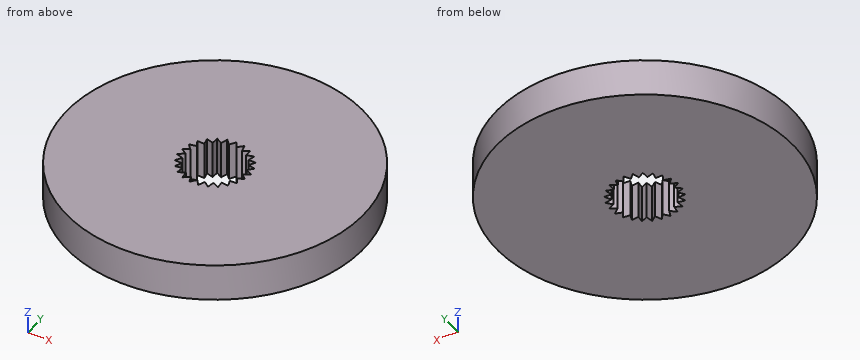
from build123d import *

# Parameters (mm, degrees)
SKETCH1_R           = 12.893401015
BOSS_EXTRUDE1_DEPTH = 3.2004


with BuildPart() as part:
    # Sketch1 → Boss-Extrude1 (new body)
    with BuildSketch(Plane.XY):
        Circle(SKETCH1_R)
        Polygon((0, 3.048), (-0.315924789, 2.500802214), (-0.758006776, 2.952241475), (-0.927923651, 2.343667613), (-1.468385199, 2.670982761), (-1.481617658, 2.039271757), (-2.086499579, 2.221896376), (-1.942216178, 1.606740957), (-2.573511517, 1.633200071), (-2.280778112, 1.073252713), (-2.898820262, 0.941883799), (-2.47603037, 0.472328054), (-3.041985468, 0.191385504), (-2.515704533, -0.158274714), (-2.99401154, -0.571138247), (-2.397307729, -0.778932499), (-2.757912856, -1.297775281), (-2.128279263, -1.350647091), (-2.348524364, -1.942868321), (-1.725523184, -1.837495558), (-1.791569449, -2.465883799), (-1.214346137, -2.208887422), (-1.122043637, -2.833958729), (-0.626867256, -2.441486766), (-0.382015696, -3.02396561), (0, -2.520678517), (0.382015696, -3.02396561), (0.626867256, -2.441486766), (1.122043637, -2.833958729), (1.214346137, -2.208887422), (1.791569449, -2.465883799), (1.725523184, -1.837495558), (2.348524364, -1.942868321), (2.128279263, -1.350647091), (2.757912856, -1.297775281), (2.397307729, -0.778932499), (2.99401154, -0.571138247), (2.515704533, -0.158274714), (3.041985468, 0.191385504), (2.47603037, 0.472328054), (2.898820262, 0.941883799), (2.280778112, 1.073252713), (2.573511517, 1.633200071), (1.942216178, 1.606740957), (2.086499579, 2.221896376), (1.481617658, 2.039271757), (1.468385199, 2.670982761), (0.927923651, 2.343667613), (0.758006776, 2.952241475), (0.315924789, 2.500802214), align=None, mode=Mode.SUBTRACT)
    extrude(amount=BOSS_EXTRUDE1_DEPTH)


solid = part.part
The model under review builds one solid part; all positions refer to its coordinate system, in mm. Give positions to 0.01 mm unless a question says otherwise; leave off trailing zeros. Loops run counter-clockwise (first coordinate to the right, second up) from the corner with the lowest first, then second, coordinate; pieces in that order, holes last. Notation, with made-up numbers: (22, 52.25) -> (65, 52.25) arc R16 ccw to (65, 80.25) -> close; hole circle Ø10 at (47, -1). An arc over 180 degrees is marked (long way). Put each result on its own line as item: value. Start each with the question number.
1. Clearance check with a flat-ended pin moving along its axis: P1, Ø1, axis at y = -2.5, z = 1.5, coming from the +X side. State where the tip first meets the part, or that it passes through.
2. We need section B-B on x = -7.25. State the section outline as (y, z) points.
3. We need section A-A on y = -4.5. State the section outline as (x, z) points.
4. Wall thickness on probe 1 along X at (y, z) = (1.5, 0.6); probe 2 along Y at (x, z) = (10, 1.8); probe 3 along Y at (x, z) = (-8.5, 2.65): over which ranges is each line inside the solid? List them lowest first.
Determined:
1. P1: x = 12.74
2. outline: (-10.66, 0) -> (10.66, 0) -> (10.66, 3.2) -> (-10.66, 3.2) -> close
3. outline: (-12.08, 0) -> (12.08, 0) -> (12.08, 3.2) -> (-12.08, 3.2) -> close
4. probe 1: -12.81 to -2.5, 2.5 to 12.81
4. probe 2: -8.14 to 8.14
4. probe 3: -9.69 to 9.69
